Part model, mm, in its own coordinate system. A direction names the side the tool comes from. Round coordinates to 2 decimals unless told otherwise and drop trailing zeros. Write each loop counter-clockwise with the first axis right and the second up, starting at its lowest first coordinate (ties: lowest second). Pieces come first, ordered by that corner, then holes. Notation, with made-up numbers: (77.5, 66) -> (94.5, 66) arc R29 cw to (94.5, 88) -> close; hole circle Ø5 at (69, -9.5). An arc over 180 degrees is marked (long way). Return JSON: item names as keys, results as strings. Group by question number.
(1) Mould opens along Y. For faces 4 (the flat face through (-83.969, -31, 40)), 5 (the flat face through (-42, 25.4, 53)), 6 (the flat face through (-52, -85.598, 42)), 7 (the cylindrical face through (-52.65, -32.62, 42.61)) say: +Y half, -Y half, draft (parallel to the pull), parting line (faces both ways), or undercut.
(2) Saw through at C-C (x = -76). List the corners of the cut face in (y, z).
(3) Drill centre lines: L1, parallel to Z at x = -52, y = -4.5; L2, parallel to Z at x = -62.5, y = -40; L3, parallel to Y at x = 5, z = 12. Where is each one in solid material? Low to high. Write a range as from..to.
(4) Saw through at A-A (y = -23). List the corners of the cut face in (x, z), plus the area to 3 significant figures.
(5) Tool access for faces 1 (the flat face through (-21.5, -42.2, 41)), 2 (the flat face through (-58, 13, 104.67)), 3 (the flat face through (-63, -42, 83.084)): list every direction of +Z, -Z, +X, -X, +Y, -Y with a clear straight run to the whole face (end or side of a thin tool).
(6) Saw through at B-B (z = 63.5). List the corners of the cut face in (x, y).
(7) Saw through at D-D (y = -64.5). List the corners of the cut face in (x, z).
(8) Drop flat-ended pins along their axis: pin 1 Ø1 at (y, z) = (-46.5, 32.5) entering from +X; pin 2 Ø10 at (y, z) = (-26, 41.5) entering from +X; pin 3 Ø5 at (y, z) = (-55, 32) entering from +X. Give the stop position or say it passes through.
from build123d import *

# Parameters (mm, degrees)
F1_DEPTH = 85.598
F3_DEPTH = 25.4
F4_R     = 11.425588
F5_DEPTH = 83.969714


with BuildPart() as f1:
    # F0 (on Front) → F1 (new body)
    with BuildSketch(Plane.XZ):
        Polygon((-83.968714, 0), (0, 0), (-43.566376, 83.084151), (-83.968714, 83.084151), align=None)
    extrude(amount=F1_DEPTH)

    # F2 (on face) → F3 (join)
    with BuildSketch(Plane(origin=(0, 0, 0), x_dir=(-1, 0, 0), z_dir=(0, 1, 0))):
        Polygon((-22.619896, 0), (83.968714, 0), (83.968714, 104.670398), (30.496623, 104.670398), align=None)
    extrude(amount=F3_DEPTH)

    # F4 (on Right) → F5 (cut, through all)
    with BuildSketch(Plane.YZ):
        with Locations((-30.146739, 53.763162)):
            Circle(F4_R)
    extrude(amount=-F5_DEPTH, mode=Mode.SUBTRACT)


solid = f1.part
Computed values:
{
 "1": {"face 4": "draft", "face 5": "+Y half", "face 6": "-Y half", "face 7": "undercut"},
 "2": {"outline": "(-85.6, 0) -> (25.4, 0) -> (25.4, 104.67) -> (0, 104.67) -> (0, 83.08) -> (-85.6, 83.08) -> close; hole circle Ø22.85 at (-30.15, 53.76)"},
 "3": {"L1": "0..83.08", "L2": "0..47.98, 59.55..83.08", "L3": "0..25.4"},
 "4": {"outline": "(-83.97, 0) -> (0, 0) -> (-23.52, 44.85) -> (-83.97, 44.85) -> close; (-83.97, 62.68) -> (-32.87, 62.68) -> (-43.57, 83.08) -> (-83.97, 83.08) -> close", "area": "4,170 mm2"},
 "5": {"face 1": "+Z, +X, -Y", "face 2": "+Z, +X, -X, +Y, -Y", "face 3": "+Z, +X, -X, -Y"},
 "6": {"outline": "(-83.97, -85.6) -> (-33.3, -85.6) -> (-33.3, -36.12) -> (-83.97, -36.12) -> close; (-83.97, -24.17) -> (-33.3, -24.17) -> (-33.3, 0) -> (-9.6, 0) -> (-9.6, 25.4) -> (-83.97, 25.4) -> close"},
 "7": {"outline": "(-83.97, 0) -> (0, 0) -> (-43.57, 83.08) -> (-83.97, 83.08) -> close"},
 "8": {"pin 1": "x = -16.78", "pin 2": "x = -19.14", "pin 3": "x = -15.47"}
}
